```python
from build123d import *

# Parameters (mm, degrees)
SKETCH1_W           = 20
SKETCH1_H           = 20
SKETCH1_W_2         = 16
SKETCH1_H_2         = 16
BOSS_EXTRUDE1_DEPTH = 212.5
SKETCH2_R           = 3
CUT_EXTRUDE1_DEPTH  = 214.673231828
SKETCH3_R           = 2.5
CUT_EXTRUDE2_DEPTH  = 214.673231828


with BuildPart() as part:
    # Sketch1 → Boss-Extrude1 (new, symmetric)
    with BuildSketch(Plane(origin=(0, 0, 0), x_dir=(0, 0, -1), z_dir=(1, 0, 0))):
        Rectangle(SKETCH1_W, SKETCH1_H)
        Rectangle(SKETCH1_W_2, SKETCH1_H_2, mode=Mode.SUBTRACT)
    extrude(amount=BOSS_EXTRUDE1_DEPTH, both=True)

    # Sketch2 → Cut-Extrude1 (cut, through all)
    with BuildSketch(Plane(origin=(0, 10, 0), x_dir=(1, 0, 0), z_dir=(0, 1, 0))):
        with Locations(Location((182.5, 0, 0), (0, 0, 270))):
            Circle(SKETCH2_R)
        with Locations(Location((202.5, 0, 0), (0, 0, 270))):
            Circle(SKETCH2_R)
    extrude(amount=-CUT_EXTRUDE1_DEPTH, mode=Mode.SUBTRACT)

    # Sketch3 → Cut-Extrude2 (cut, through all)
    with BuildSketch(Plane(origin=(0, 10, 0), x_dir=(1, 0, 0), z_dir=(0, 1, 0))):
        with Locations(Location((-202.5, 0, 0), (0, 0, 270))):
            Circle(SKETCH3_R)
        with Locations(Location((-182.5, 0, 0), (0, 0, 270))):
            Circle(SKETCH3_R)
    extrude(amount=-CUT_EXTRUDE2_DEPTH, mode=Mode.SUBTRACT)


solid = part.part
```
CAD build for the part. Positions are in the model's coordinates, mm. A direction names the side the tool comes from. Round coordinates to 2 decimals unless told otherwise and drop trailing zeros. Order: outer loops, then holes, each group sorted by start corner. A loop starts at its lowest first (then second) coordinate and runs counter-clockwise, first axis right, second up.
Item 1: Saw through at A-A on x = -108. Write the cut outline in (y, z), then the cut area to 3 significant figures.
Item 2: Probe line 1 along X through (y, z) = (-9.25, 0); line 2 along Z through (x, y) = (153, 7.75). List the from-to ranges inside material, lowest first.
Item 3: Saw through at B-B on y = 3.5. Write the cut outline in (x, z).
Item 4: Tool access for faces 1 (the face through (-212.5, 0, 9)), 2 (the face through (3, 8, 0)): list every direction of +Z, -Z, +X, -X, +Y, -Y with a clear straight run to the whole face (end or side of a thin tool).
Item 5: Pin check, flat tip, straight feed: pin 1 (4 mm diameter, centred on y = 6.5, z = -5.5, fed in from -X). Stop position of the tip, or through.
Item 6: Mould opens along Z. For faces 3 (the face through (3, 0, 10)), 4 (the face through (3, 10, 0)), 5 (the face through (3, -8, 0)) say: pulls with the +Z half, pulls with the -Z half, needs draft (parallel to the pull), parting line crosses it, or undercut.
Reported:
1. outline: (-10, -10) - (10, -10) - (10, 10) - (-10, 10) - close; hole (-8, -8) - (8, -8) - (8, 8) - (-8, 8) - close
1. area: 144 mm2
2. line 1: x = -212.5 to -205, -200 to -185, -180 to 179.5, 185.5 to 199.5, 205.5 to 212.5
2. line 2: z = -10 to -8, 8 to 10
3. outline: (-212.5, -10) - (212.5, -10) - (212.5, -8) - (-212.5, -8) - close; (-212.5, 8) - (212.5, 8) - (212.5, 10) - (-212.5, 10) - close
4. face 1: +Z, -Z, -X, +Y, -Y
4. face 2: +X, -X
5. pin 1: stops at x = -212.5
6. face 3: pulls with the +Z half
6. face 4: needs draft
6. face 5: undercut
